Autodesk Inventor part; units mm, degrees
ref_plane "YZ Plane" through (0, 0, 0) normal (1, 0, 0) x (0, 1, 0)
ref_plane "XZ Plane" through (0, 0, 0) normal (0, 1, 0) x (-1, 0, 0)
ref_plane "XY Plane" through (0, 0, 0) normal (0, 0, 1) x (1, 0, 0)
sketch "Sketch1" plane through (0, 0, 0) normal (0, 0, 1) x (1, 0, 0)
  line L0 (0, 0) -> (-76.2, 0)
  line L1 (-76.2, 0) -> (-76.2, -25.4)
  line L2 (-76.2, -25.4) -> (0, -25.4)
  line L3 (0, -25.4) -> (0, 0)
  circle A0 centre (-50.8, -9.525) radius 1.27
  circle A1 centre (-25.4, -9.525) radius 1.27
  dimension "d0" = 76.2
  dimension "d1" = 25.4
  dimension "d2" = 25.4
  dimension "d3" = 25.4
  dimension "d4" = 2.54
  dimension "d5" = 9.525
  dimension "d6" = 9.525
extrude "Extrusion1" add sketch "Sketch1" along normal blind 12.7
sketch "Sketch2" plane through (-76.2, 0, 0) normal (0, 1, 0) x (1, 0, 0)
  circle A0 centre (31.75, -6.35) radius 3.175
  circle A1 centre (44.45, -6.35) radius 3.175
  line L0 (0, 0) -> (76.2, 0)
  line L1 (0, 0) -> (0, -12.7)
  line L2 (76.2, 0) -> (76.2, -12.7)
  dimension "d9" = 6.35
  dimension "d10" = 6.35
  dimension "d11" = 6.35
  dimension "d12" = 6.35
  dimension "d13" = 31.75
  dimension "d14" = 31.75
extrude "Extrusion2" cut sketch "Sketch2" against normal blind 6.35
sketch "Sketch3" plane through (-76.2, -25.4, 0) normal (0, -1, 0) x (1, 0, 0)
  circle A0 centre (38.1, 6.35) radius 3.175
  line L0 (76.2, 0) -> (76.2, 12.7)
  line L1 (0, 0) -> (76.2, 0)
  dimension "d17" = 6.35
  dimension "d18" = 38.1
  dimension "d19" = 6.35
extrude "Extrusion3" cut sketch "Sketch3" against normal blind 6.35
properties part number "solenoid valve" material "PC/ABS Plastic"
Work out the finished part from the listing and answer in its coordinate system (mm). A direction names the side the tool comes from. Round coordinates to 2 decimals unless told otherwise and drop trailing zeros. Order: outer loops, then holes, each group sorted by start corner. A loop starts at its lowest first (then second) coordinate and runs counter-clockwise, first axis right, second up. Notation, with made-up numbers: M 6,16.5 L 39,16.5 A22 cw 39,23.5 Z; hole C 70,42 d3. An arc over 180 degrees is marked long. Put each result on its own line as item: value. Start each with the question number.
Q1. Flat-ended cylindrical pins translate along their axes: pin 1 (1.9 mm diameter, centred on x = -32, z = 8, fed in from +Y); pin 2 (2 mm diameter, centred on x = -50.8, y = -9.525, fed in from -Z). Find the tip coordinate at first contact, or state that the pin passes through.
Q2. Section D-D, the plane x = -31.75 is taken. Write down the section's boundary in (y, z) (3 decimals), and give its area (3 significant figures).
Q3. Section A-A, the plane x = -50.8 is taken. Write down the section's boundary in (y, z) (3 decimals), and give its area (3 significant figures).
Q4. For a pull along Z with two mould halves and no side action, classify faces 4 (the flat face through (0, -13, 6)), 5 (the flat face through (-44, -6.35, 6)), 6 (the flat face through (-39, -13, 12.7)) as pulls with the +Z half, pulls with the -Z half, needs draft (parallel to the pull), parting line crosses it, or undercut.
Q5. A tool of negligible diameter and unlimited length cuts with its end or side. For faces 1 (the flat face through (-32, -6.35, 6)), 2 (the cylindrical face through (-24.81, -8.4, 6.26)), 3 (the cylindrical face through (-40.44, -22.269, 8.496)), from which of +Z, -Z, +X, -X, +Y, -Y can it reach the whole face along a straight path? Write none if from no direction.
Q6. Section B-B, the plane y = -20.5 is taken. Write down the section's boundary in (x, z) (3 decimals), and give its area (3 significant figures).
Q7. Straight lines are drawn through the part: L1, parallel to Z at x = -44.45, y = -4 (3 decimals); L2, parallel to Y at x = -51, z = 2.75; L3, parallel to X at y = -1.75, z = 4.5. For each, find the intervals that lie inside material, in ascending order. Write a range as [from, to].
Q8. Section C-C, the plane z = 8.5 is taken. Write down the section's boundary in (x, y) (3 decimals).
Findings below:
1. pin 1: stops at y = -6.35
1. pin 2: passes through
2. outline: M -25.4,0 L 0,0 L 0,3.175 L -6.35,3.175 L -6.35,9.525 L 0,9.525 L 0,12.7 L -25.4,12.7 Z
2. area: 282 mm^2
3. outline: M -25.4,0 L -10.795,0 L -10.795,12.7 L -25.4,12.7 Z; M -8.255,0 L 0,0 L 0,12.7 L -8.255,12.7 Z
3. area: 290 mm^2
4. face 4: needs draft
4. face 5: undercut
4. face 6: pulls with the +Z half
5. face 1: +Y
5. face 2: +Z, -Z
5. face 3: -Y
6. outline: M -76.2,0 L 0,0 L 0,12.7 L -76.2,12.7 Z; hole C -38.1,6.35 d6.35
6. area: 936 mm^2
7. L1: z = [0, 3.175], [9.525, 12.7]
7. L2: y = [-25.4, -10.78], [-8.27, 0]
7. L3: x = [-76.2, -47.03], [-41.87, -34.33], [-29.17, 0]
8. outline: M -76.2,-25.4 L -40.436,-25.4 L -40.436,-19.05 L -35.764,-19.05 L -35.764,-25.4 L 0,-25.4 L 0,0 L -29.414,0 L -29.414,-6.35 L -34.086,-6.35 L -34.086,0 L -42.114,0 L -42.114,-6.35 L -46.786,-6.35 L -46.786,0 L -76.2,0 Z; hole C -50.8,-9.525 d2.54; hole C -25.4,-9.525 d2.54
